Build history of the part. All positions in model axes, mm. A direction names the side the tool comes from. Round coordinates to 2 decimals unless told otherwise and drop trailing zeros. Loops run counter-clockwise (first coordinate to the right, second up) from the corner with the lowest first, then second, coordinate; pieces in that order, holes last.
from build123d import *


# Read off the part's stored shape, not the designer's step: M10x0.75 Machine Threads Stud1
with BuildPart() as part:
    # Sketch1 → Revolve2 (revolve)
    with BuildSketch(Plane.XY, mode=Mode.PRIVATE) as revolve2_sk:
        Polygon((0, 0), (0, 150), (5, 150), (5, -50), (0, -50), (-10, -40), (-10, -10), align=None)
    revolve(revolve2_sk.sketch.rotate(Axis((5, 0, 0), (0, 1, 0)), 270), axis=Axis((5, 0, 0), (0, 1, 0)))

    # M10x0.75 Machine Threads Stud1 outline → M10x0.75 Machine Threads Stud1 (revolve, cut)
    with BuildSketch(Plane(origin=(5, 0, 0), x_dir=(1, 0, 0), z_dir=(0, 0, 1))):
        Polygon((5, 150), (4.54, 150), (4.7565, 149.7835), (4.7565, 0), (5, 0), align=None)
    revolve(axis=Axis((5, 0, 0), (0, 1, 0)), mode=Mode.SUBTRACT)


solid = part.part
(1) Probe line 1 (X direction, y = 105, z = 0.25); line 2 (X direction, y = -32, z = 0); line 3 (Z direction, x = 3.5, y = 7). List the from-to ranges inside material, lowest first.
Responses:
line 1: x = 0.25 to 9.75
line 2: x = -10 to 20
line 3: z = -4.51 to 4.51
(2) Slice it at A-A on z = 0. List the corners of the cut face in (x, y), plus the area to 3 significant figures.
Responses:
outline: (-10, -40) - (0, -50) - (10, -50) - (20, -40) - (20, -10) - (10, 0) - (9.76, 0) - (9.76, 149.78) - (9.54, 150) - (0.46, 150) - (0.24, 149.78) - (0.24, 0) - (0, 0) - (-10, -10) - close
area: 2,730 mm2
(3) Slice it at B-B on x = 5. List the corners of the cut face in (y, z), plus the area to 3 significant figures.
Responses:
outline: (-50, -5) - (-40, -15) - (-10, -15) - (0, -5) - (0, -4.76) - (149.78, -4.76) - (150, -4.54) - (150, 4.54) - (149.78, 4.76) - (0, 4.76) - (0, 5) - (-10, 15) - (-40, 15) - (-50, 5) - close
area: 2,730 mm2
(4) Which spindle directions (+Z, -Z, +X, -X, +Y, -Y) get a long thin tool onto all of the face, cutting with end or side? Do faces 1 (the face through (3.31, -49.37, -5.37)), 2 (the face through (7.56, 73.84, -4.01)). Say none if no direction does.
Responses:
face 1: -Y
face 2: +Y
(5) Slice it at C-C on y = 84.5. List the corners of the cut face in (x, z).
Responses:
outline: circle Ø9.51 at (5, 0)
(6) Pin check, flat tips, straight feed: P1, Ø12, axis at x = -4, y = 34, coming from the +Z side; P2, Ø6, axis at x = -5, z = 11, coming from the -Y side; P3, Ø8, axis at x = -2.5, z = 10, coming from the -Y side. Stop position of each tip, or through.
Responses:
P1: stops at z = 3.69
P2: stops at y = -43.13
P3: stops at y = -46.5
